```python
from build123d import *

# Parameters (mm, degrees)
SKETCH1_W           = 151
SKETCH1_H           = 255
BOSS_EXTRUDE1_DEPTH = 5
SKETCH2_W           = 49.486524855
SKETCH2_H           = 131.582895272
CUT_EXTRUDE1_DEPTH  = 5
SKETCH3_W           = 30.1
SKETCH3_H           = 5.1
SKETCH3_W_2         = 20.1
CUT_EXTRUDE2_DEPTH  = 5
SKETCH4_R           = 2
CUT_EXTRUDE3_DEPTH  = 5
SKETCH5_R           = 4
SKETCH5_R_2         = 2
BOSS_EXTRUDE2_DEPTH = 5
SKETCH6_W           = 24
SKETCH6_H           = 30
CUT_EXTRUDE4_DEPTH  = 5
SKETCH7_R           = 2
CUT_EXTRUDE5_DEPTH  = 10


with BuildPart() as part:
    # Sketch1 → Boss-Extrude1 (new body)
    with BuildSketch(Plane.XY):
        Rectangle(SKETCH1_W, SKETCH1_H)
    extrude(amount=BOSS_EXTRUDE1_DEPTH)

    # Sketch2 → Cut-Extrude1 (cut)
    with BuildSketch(Plane.XY.offset(5)):
        with Locations((-50.756737573, -61.708552364)):
            Rectangle(SKETCH2_W, SKETCH2_H)
    extrude(amount=-CUT_EXTRUDE1_DEPTH, mode=Mode.SUBTRACT)

    # Sketch3 → Cut-Extrude2 (cut)
    with BuildSketch(Plane.XY.offset(5)):
        with Locations((-40.45, 124.95)):
            Rectangle(SKETCH3_W, SKETCH3_H)
        with Locations((40.55, 124.95)):
            Rectangle(SKETCH3_W, SKETCH3_H)
        with Locations((-40.440248728, 55.95)):
            Rectangle(SKETCH3_W, SKETCH3_H)
        with Locations((20.55, 55.95)):
            Rectangle(SKETCH3_W, SKETCH3_H)
        with Locations((30.55, 6.95)):
            Rectangle(SKETCH3_W, SKETCH3_H)
        with Locations((6.55, -58.05)):
            Rectangle(SKETCH3_W_2, SKETCH3_H)
        with Locations((24.55, -124.95)):
            Rectangle(SKETCH3_W, SKETCH3_H)
    extrude(amount=-CUT_EXTRUDE2_DEPTH, mode=Mode.SUBTRACT)

    # Sketch4 → Cut-Extrude3 (cut)
    with BuildSketch(Plane.XY.offset(5)):
        with Locations((0, 125)):
            Circle(SKETCH4_R)
        with Locations((-2.045010771, 56)):
            Circle(SKETCH4_R)
        with Locations((60.936739195, 7)):
            Circle(SKETCH4_R)
        with Locations((-12.405611853, -58)):
            Circle(SKETCH4_R)
    extrude(amount=-CUT_EXTRUDE3_DEPTH, mode=Mode.SUBTRACT)

    # Sketch5 → Boss-Extrude2 (add)
    with BuildSketch(Plane.XY.offset(5)):
        with Locations((0, 125)):
            Circle(SKETCH5_R)
        with Locations((0, 125)):
            Circle(SKETCH5_R_2, mode=Mode.SUBTRACT)
    extrude(amount=-BOSS_EXTRUDE2_DEPTH)

    # Sketch6 → Cut-Extrude4 (cut)
    with BuildSketch(Plane.XY.offset(5)):
        with Locations((49.941975166, 31.5)):
            Rectangle(SKETCH6_W, SKETCH6_H)
    extrude(amount=-CUT_EXTRUDE4_DEPTH, mode=Mode.SUBTRACT)

    # Sketch7 → Cut-Extrude5 (cut)
    with BuildSketch(Plane.XY.offset(5)):
        with Locations((68.5, 103.580315126)):
            Circle(SKETCH7_R)
        with Locations((5.5, 80.580315126)):
            Circle(SKETCH7_R)
        with Locations((5.5, 103.580315126)):
            Circle(SKETCH7_R)
        with Locations((68.5, 80.580315126)):
            Circle(SKETCH7_R)
    extrude(amount=-CUT_EXTRUDE5_DEPTH, mode=Mode.SUBTRACT)


solid = part.part
```
Geometry check sheet. Reference: the model listing, model coordinates, mm. A direction names the side the tool comes from. Give positions to 0.01 mm unless a question says otherwise; leave off trailing zeros. Write each loop counter-clockwise with the first axis right and the second up, starting at its lowest first coordinate (ties: lowest second). Pieces come first, ordered by that corner, then holes.
1) Gauge pin test, flat ends, axial feed: pin 1 (2.5 mm diameter, centred on x = -17, z = 2.5, fed in from +Y); pin 2 (2 mm diameter, centred on x = 48.5, z = 2, fed in from +Y). Record the tip position at first contact, or that the pin passes through.
2) Material ranges on L1, parallel to X at y = 103.5, z = 4.6; L2, parallel to Y at x = 15, z = 0.85; L3, parallel to Y at x = -27.5, z = 2.4, recorded low to high.
3) Section check A-A, the plane y = 33. Record the boundary of the cut face in (x, z), and give its area (3 significant figures).
4) Section check B-B, the plane y = -72. Record the boundary of the cut face in (x, z), and give its area (3 significant figures).
5) Section check C-C, the plane z = 2.45. State how many separate pieces and enclosed holes the cut face has, and give its area (3 significant figures).
6) Access from +Z, -Z, +X, -X, +Y, -Y to the whole of each face (thin tool, end or side, straight path). Record for faces 1 (the flat face through (-26.013, -63, 3)), 2 (the flat face through (-25.4, 125, 3)), 3 (the flat face through (14, 127.5, 2)), 4 (the flat face through (50, 16.5, 3)).
7) Release check for a two-part mould opening along X. For faces 5 (the flat face through (-25.39, 56, 3)), 6 (the flat face through (75.5, -2, 2)), 7 (the flat face through (-41, 58.5, 3)), 8 (the flat face through (-75.5, 65, 2)) record: pulls with the +X half, pulls with the -X half, needs draft (parallel to the pull), parting line crosses it, or undercut.
Computed:
1. pin 1: stops at y = 127.5
1. pin 2: stops at y = 122.4
2. L1: x = -75.5 to 3.5, 7.5 to 66.5, 70.5 to 75.5
2. L2: y = -122.4 to -60.6, -55.5 to 53.4, 58.5 to 127.5
2. L3: y = 4.08 to 53.4, 58.5 to 122.4
3. outline: (-75.5, 0) - (37.94, 0) - (37.94, 5) - (-75.5, 5) - close; (61.94, 0) - (75.5, 0) - (75.5, 5) - (61.94, 5) - close
3. area: 635 mm2
4. outline: (-26.01, 0) - (75.5, 0) - (75.5, 5) - (-26.01, 5) - close
4. area: 508 mm2
5. separate pieces: 1
5. enclosed holes: 13
5. area: 30,200 mm2
6. face 1: +Z, -Z, -X, -Y
6. face 2: +Z, -Z, +Y
6. face 3: +Z, -Z, +X, +Y
6. face 4: +Z, -Z
7. face 5: undercut
7. face 6: pulls with the +X half
7. face 7: undercut
7. face 8: pulls with the -X half
